Job drawing, mm, ordinate dimensions from the low corner. One solid piece. Coordinates: 2 decimals unless noted, no trailing zeros. Loops run counter-clockwise (first coordinate to the right, second up) from the corner with the lowest first, then second, coordinate; pieces in that order, holes last. Notation, with made-up numbers: M 28,-2 L 49,-2 A19 cw 49,15 Z; hole C 5,6.5 d10. An arc over 180 degrees is marked long. Answer as a JSON object with one key per item and string values. Group by question number.
1. Drop flat-ended pins along their axis: pin 1 Ø1.8 at (y, z) = (14, 22.5) entering from -X; pin 2 Ø2 at (x, z) = (25, 51.5) entering from -Y; pin 3 Ø0.8 at (x, z) = (1.5, 30) entering from -Y; pin 4 Ø5 at (x, z) = (58, 48.5) entering from -Y. Give the stop position or say it passes through.
2. Saw through at B-B on z = 34.5. Write the cut outline in (x, y).
3. Saw through at C-C on y = 4.25. Write the cut outline in (x, z).
4. Saw through at A-A on y = 13.25. Write the cut outline in (x, z), then the cut area to 3 significant figures.
5. Mould opens along X. For the marked faces 1 and 2 say: released by +X, released by -X, zero draft, split by the parting line, or undercut.
6. Drill centre lines: L1, parallel to X at y = 12.5, z = 49.5; L2, parallel to X at y = 20.5, z = 15.5; L3, parallel to X at y = 4, z = 53.5 (1 decimal). Where is each one in solid material? Low to high.
7. Saw through at D-D on y = 9. Write the cut outline in (x, z), then the cut area to 3 significant figures.
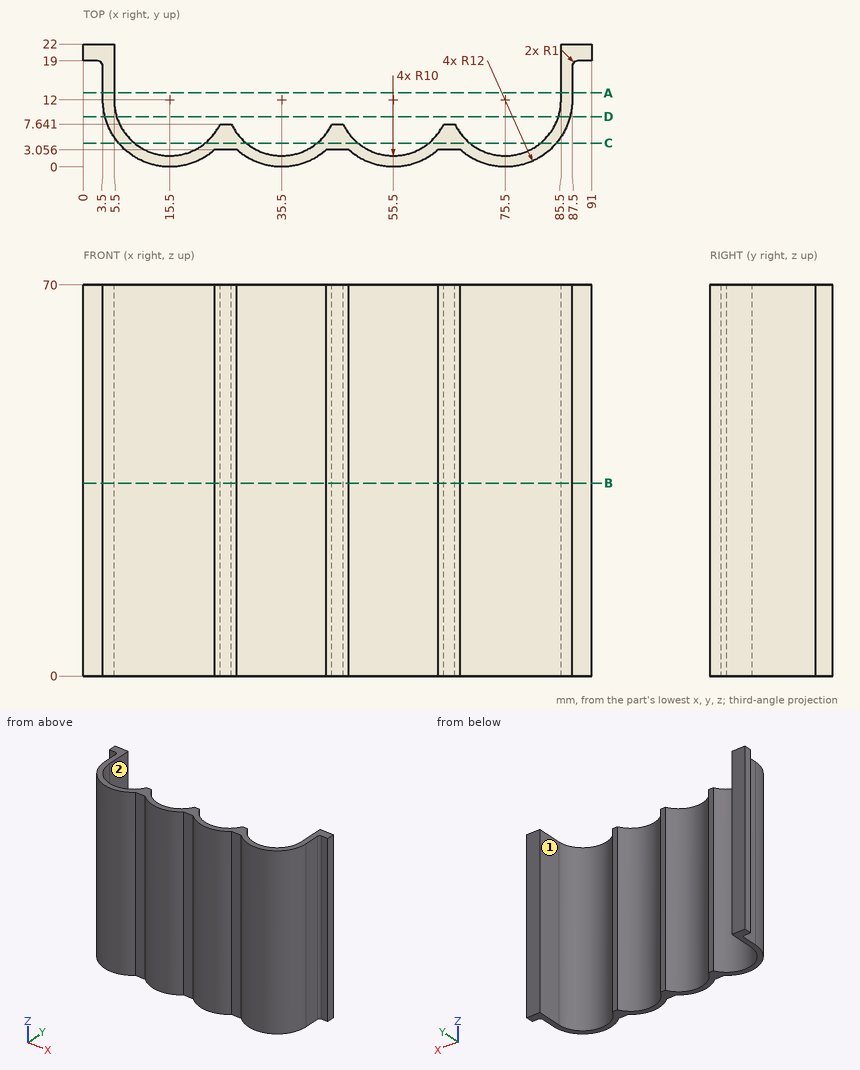
Outcome:
{
 "1": {"pin 1": "stops at x = 3.5", "pin 2": "stops at y = 3.06", "pin 3": "stops at y = 19", "pin 4": "stops at y = 0"},
 "2": {"outline": "M 0,19 L 2.5,19 A1 cw 3.5,18 L 3.5,12 A12 ccw 23.5,3.06 L 27.5,3.06 A12 ccw 43.5,3.06 L 47.5,3.06 A12 ccw 63.5,3.06 L 67.5,3.06 A12 ccw 87.5,12 L 87.5,18 A1 cw 88.5,19 L 91,19 L 91,22 L 85.5,22 L 85.5,12 A10 cw 66.5,7.64 L 64.5,7.64 A10 cw 46.5,7.64 L 44.5,7.64 A10 cw 26.5,7.64 L 24.5,7.64 A10 cw 5.5,12 L 5.5,22 L 0,22 Z"},
 "3": {"outline": "M 6.34,0 L 9.18,0 L 9.18,70 L 6.34,70 Z; M 21.82,0 L 29.18,0 L 29.18,70 L 21.82,70 Z; M 41.82,0 L 49.18,0 L 49.18,70 L 41.82,70 Z; M 61.82,0 L 69.18,0 L 69.18,70 L 61.82,70 Z; M 81.82,0 L 84.66,0 L 84.66,70 L 81.82,70 Z"},
 "4": {"outline": "M 3.5,0 L 5.5,0 L 5.5,70 L 3.5,70 Z; M 85.5,0 L 87.5,0 L 87.5,70 L 85.5,70 Z", "area": "280 mm²"},
 "5": {"face 1": "undercut", "face 2": "undercut"},
 "6": {"L1": "x = 3.5 to 5.5, 85.5 to 87.5", "L2": "x = 0 to 5.5, 85.5 to 91", "L3": "x = 6.6 to 9.5, 21.5 to 29.5, 41.5 to 49.5, 61.5 to 69.5, 81.5 to 84.4"},
 "7": {"outline": "M 3.88,0 L 5.96,0 L 5.96,70 L 3.88,70 Z; M 85.04,0 L 87.12,0 L 87.12,70 L 85.04,70 Z", "area": "291 mm²"}
}
